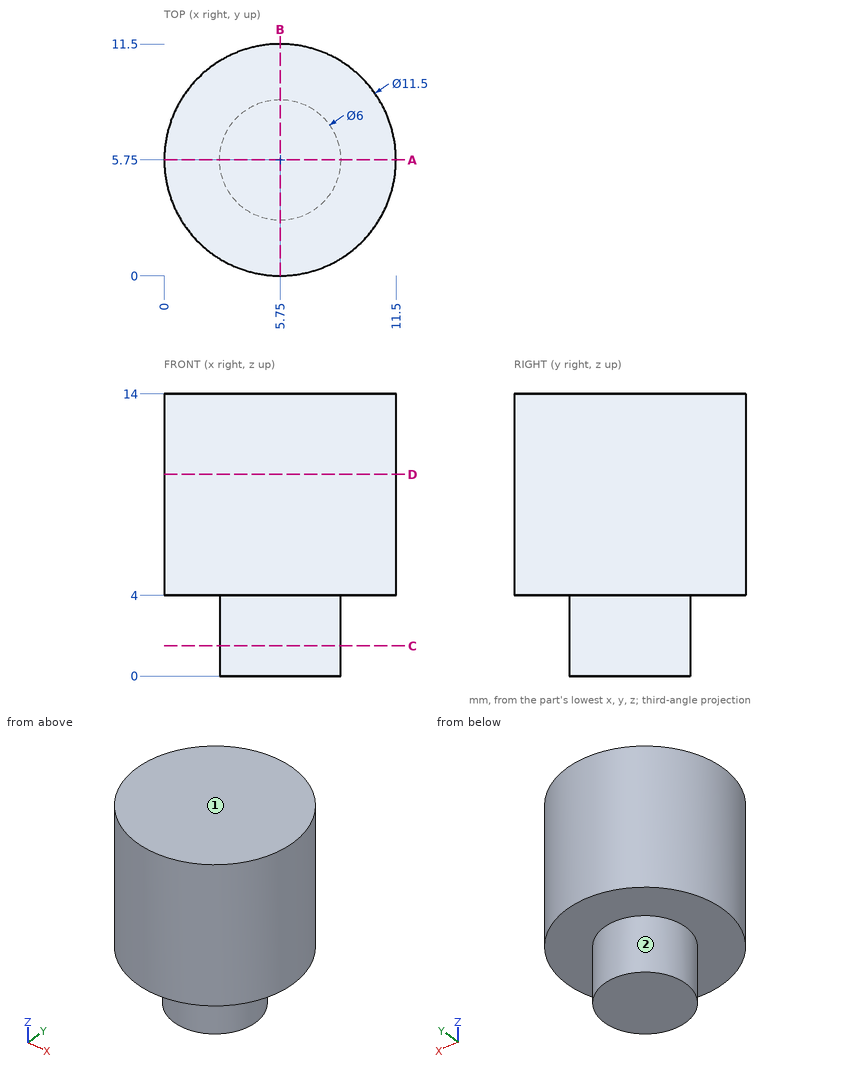
Drawing for the job (mm, zero at the part's lowest x, y, z). A direction names the side the tool comes from. Round coordinates to 2 decimals unless told otherwise and drop trailing zeros. Order: outer loops, then holes, each group sorted by start corner. A loop starts at its lowest first (then second) coordinate and runs counter-clockwise, first axis right, second up. Notation, with made-up numbers: (-1.5, 50.25) -> (45.5, 50.25) arc R11 ccw to (45.5, 56.25) -> close; hole circle Ø3 at (-20.75, 82.25). An arc over 180 degrees is marked (long way). Write item = value, one per line. Start each with the question number.
(1) Which spindle directions (+Z, -Z, +X, -X, +Y, -Y) get a long thin tool onto all of the face, cutting with end or side? Do the marked faces 1 and 2. Say none if no direction does.
(2) Cut at D-D, the plane z = 10. List the corners of the cut face in (x, y), then the cut area to 3 significant figures.
(3) Cut at A-A, the plane y = 5.75. List the corners of the cut face in (x, z).
(4) Cut at C-C, the plane z = 1.5. List the corners of the cut face in (x, y).
(5) Pin check, flat tips, straight feed: P1, Ø2, axis at y = 4.5, z = 5.5, coming from the +X side; P2, Ø4, axis at x = 7.5, z = 2.5, coming from the -Y side. Stop position of each tip, or through.
(6) Probe line 1 (Z direction, x = 3, y = 10.5); line 2 (Y direction, x = 6, z = 11.5); line 3 (X direction, y = 8.75, z = 5.25). List the from-to ranges inside material, lowest first. Write a range as [from, to].
Model answer:
q1.face_1 = +Z, +X, -X, +Y, -Y
q1.face_2 = -Z
q2.outline = circle Ø11.5 at (5.75, 5.75)
q2.area = 104 mm2
q3.outline = (0, 4) -> (2.75, 4) -> (2.75, 0) -> (8.75, 0) -> (8.75, 4) -> (11.5, 4) -> (11.5, 14) -> (0, 14) -> close
q4.outline = circle Ø6 at (5.75, 5.75)
q5.P1 = 11.49
q5.P2 = 0.02
q6.line_1 = [4, 14]
q6.line_2 = [0.01, 11.49]
q6.line_3 = [0.84, 10.66]
